Can you work these out from the model? Positions are in its coordinate system, mm. A direction names the side the tool comes from. Give positions to 0.01 mm unless a question says otherwise; leave off trailing zeros. Loops run counter-clockwise (first coordinate to the right, second up) from the corner with the lowest first, then second, coordinate; pieces in that order, holes last. Notation, with made-up numbers: (30, 84) - (60, 84) arc R21 cw to (60, 97) - close; hole circle Ø1 at (-14, 0). An arc over 180 degrees is marked (long way). Use a Markdown table: item, result. Add a question column.
```python
from build123d import *

# Parameters (mm, degrees)
SKETCH_1_W      = 89
SKETCH_1_H      = 97
SKETCH_1_R      = 1
EXTRUDE_1_DEPTH = 1.2
SKETCH_2_R      = 3.15
EXTRUDE_2_DEPTH = 4.4
SKETCH_3_W      = 36
SKETCH_3_H      = 97
EXTRUDE_3_DEPTH = 4.5
SKETCH_4_W      = 1.5
SKETCH_4_H      = 8.5
EXTRUDE_5_DEPTH = 97
SKETCH_5_W      = 13.6
SKETCH_5_H      = 13.1
EXTRUDE_6_DEPTH = 7.3
SKETCH_6_W      = 17.7
SKETCH_6_H      = 15.2
EXTRUDE_7_DEPTH = 14.8
SKETCH_7_W      = 11.5
SKETCH_7_H      = 9.5
EXTRUDE_8_DEPTH = 7.38


with BuildPart() as part:
    # 草图1 → 凸台-拉伸1 (new body)
    with BuildSketch(Plane(origin=(0, 0, 0), x_dir=(1, 0, 0), z_dir=(0, 1, 0))):
        with Locations((-44.5, 48.5)):
            Rectangle(SKETCH_1_W, SKETCH_1_H)
        with Locations((-7, 94.5)):
            Circle(SKETCH_1_R, mode=Mode.SUBTRACT)
        with Locations((-7, 2.5)):
            Circle(SKETCH_1_R, mode=Mode.SUBTRACT)
        with Locations((-56, 91.4)):
            Circle(SKETCH_1_R, mode=Mode.SUBTRACT)
        with Locations((-27.5, 91.4)):
            Circle(SKETCH_1_R, mode=Mode.SUBTRACT)
    extrude(amount=EXTRUDE_1_DEPTH)

    # 草图2 → 凸台-拉伸2 (add)
    with BuildSketch(Plane(origin=(0, 1.2, 0), x_dir=(1, 0, 0), z_dir=(0, 1, 0))):
        with Locations((-51, 81)):
            Circle(SKETCH_2_R)
    extrude(amount=EXTRUDE_2_DEPTH)

    # 草图3 → 凸台-拉伸3 (add)
    with BuildSketch(Plane.XZ):
        with Locations((-42, -48.5)):
            Rectangle(SKETCH_3_W, SKETCH_3_H)
    extrude(amount=EXTRUDE_3_DEPTH)

    # 草图4 → 凸台-拉伸5 (add, through all)
    with BuildSketch(Plane(origin=(0, 0, -97), x_dir=(-1, 0, 0), z_dir=(0, 0, -1))):
        with Locations((26.75, -8.75)):
            Rectangle(SKETCH_4_W, SKETCH_4_H)
        with Locations((32.75, -8.75)):
            Rectangle(SKETCH_4_W, SKETCH_4_H)
        with Locations((38.75, -8.75)):
            Rectangle(SKETCH_4_W, SKETCH_4_H)
        with Locations((44.75, -8.75)):
            Rectangle(SKETCH_4_W, SKETCH_4_H)
        with Locations((50.75, -8.75)):
            Rectangle(SKETCH_4_W, SKETCH_4_H)
        with Locations((56.75, -8.75)):
            Rectangle(SKETCH_4_W, SKETCH_4_H)
    extrude(amount=-EXTRUDE_5_DEPTH)

    # 草图5 → 凸台-拉伸6 (add)
    with BuildSketch(Plane.XZ):
        with Locations((-82.2, -63.4)):
            Rectangle(SKETCH_5_W, SKETCH_5_H)
    extrude(amount=EXTRUDE_6_DEPTH)

    # 草图6 → 凸台-拉伸7 (add)
    with BuildSketch(Plane.XZ):
        with Locations((-80.15, -97.01)):
            Rectangle(SKETCH_6_W, SKETCH_6_H)
    extrude(amount=EXTRUDE_7_DEPTH)

    # 草图7 → 凸台-拉伸8 (add)
    with BuildSketch(Plane.XZ):
        with Locations((-83.25, -10.48)):
            Rectangle(SKETCH_7_W, SKETCH_7_H)
    extrude(amount=EXTRUDE_8_DEPTH)


solid = part.part
```
1. Will these pins go through, and if not, where does the flat tip stop? P1, Ø12, axis at x = -42.5, z = -33.5, coming from the -Y side; P2, Ø3, axis at x = -74.5, z = -20.5, coming from the -Y side; P3, Ø9.5, axis at y = -6.5, z = -43.5, coming from the -X side; P4, Ø1, axis at x = -36, y = -3.5, coming from the +Z side.
2. On a 3-axis mill with a long thin cutter (end or side, diameter ignored), from which of +Z, -Z, +X, -X, +Y, -Y can I reach the whole of each face in a straight line? I mean faces 1 (the face through (-83, -4, -15.23)), 2 (the face through (-42, -4.5, -48)), 3 (the face through (-75.4, -4, -63)). Say none if no direction works.
3. Please list where these lines run through material, in increasing order: line 1 along X through (y, z) = (0.55, -91.4); line 2 along Z through (x, y) = (-78.5, -0.25); line 3 along X through (y, z) = (-12.25, -33). Write a range as [from, to].
4. Suppose I cut it at C-C (x = -53). List the corners of the cut face in (y, z) for me, and give its area (3 significant figures).
5. Suppose I cut it at D-D (y = 3.25). List the corners of the cut face in (x, z) for me.
6. Suppose I cut it at A-A (y = -11). List the corners of the cut face in (x, z) for me, and give its area (3 significant figures).
7. If we mould it in two halves opening along Z, with no side actions, what happens to faces 4 (the face through (-82, -4, -69.95)), 5 (the face through (-45, -3, 0)), 6 (the face through (-75, 0, -49)), 7 (the face through (-77.5, -4, -11))? For each: released by +Z, released by -Z, zero draft, split by the parting line, or undercut.
Results below:
| question | item | result |
|---|---|---|
| 1 | P1 | y = -13 |
| 1 | P2 | y = 0 |
| 1 | P3 | x = -60 |
| 1 | P4 | z = 0 |
| 2 | face 1 | -X, -Y |
| 2 | face 2 | +Z, -Z, -Y |
| 2 | face 3 | +Z, -Y |
| 3 | line 1 | [-89, -57], [-55, -28.5], [-26.5, 0] |
| 3 | line 2 | [-104.61, -89.41], [-69.95, -56.85], [-15.23, -5.73] |
| 3 | line 3 | [-57.5, -56], [-51.5, -50], [-45.5, -44], [-39.5, -38], [-33.5, -32], [-27.5, -26] |
| 4 | outline | (-4.5, -97) - (1.2, -97) - (1.2, -83.43) - (5.6, -83.43) - (5.6, -78.57) - (1.2, -78.57) - (1.2, 0) - (-4.5, 0) - close |
| 4 | area | 574 mm² |
| 5 | outline | circle Ø6.3 at (-51, -81) |
| 6 | outline | (-89, -104.61) - (-71.3, -104.61) - (-71.3, -89.41) - (-89, -89.41) - close; (-57.5, -97) - (-56, -97) - (-56, 0) - (-57.5, 0) - close; (-51.5, -97) - (-50, -97) - (-50, 0) - (-51.5, 0) - close; (-45.5, -97) - (-44, -97) - (-44, 0) - (-45.5, 0) - close; (-39.5, -97) - (-38, -97) - (-38, 0) - (-39.5, 0) - close; (-33.5, -97) - (-32, -97) - (-32, 0) - (-33.5, 0) - close; (-27.5, -97) - (-26, -97) - (-26, 0) - (-27.5, 0) - close |
| 6 | area | 1,140 mm² |
| 7 | face 4 | undercut |
| 7 | face 5 | released by +Z |
| 7 | face 6 | undercut |
| 7 | face 7 | zero draft |
